Drawing for the job (mm, zero at the part's lowest x, y, z). A direction names the side the tool comes from. Round coordinates to 2 decimals unless told otherwise and drop trailing zeros. Loops run counter-clockwise (first coordinate to the right, second up) from the corner with the lowest first, then second, coordinate; pieces in that order, holes last.
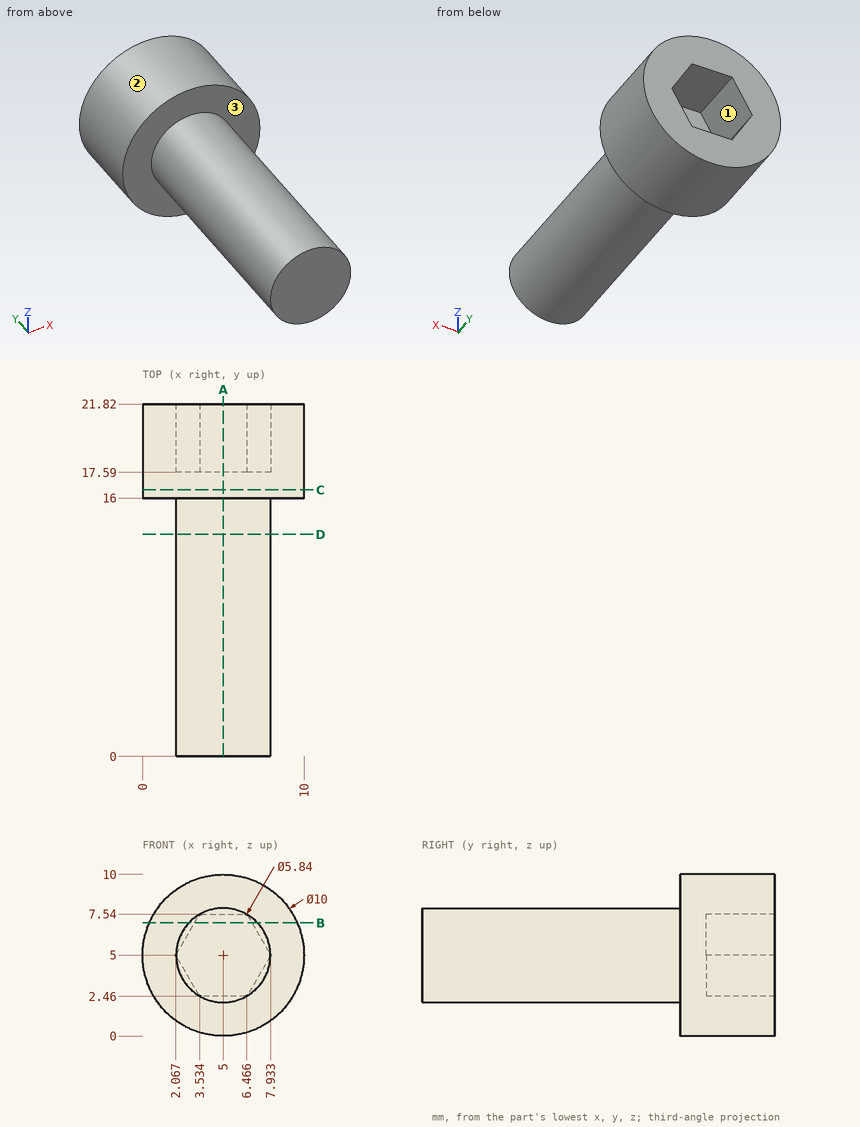
Q1. Probe line 1 (Z direction, x = 5, y = 20); line 2 (Y direction, x = 3, z = 9); line 3 (Y direction, x = 4.5, z = 3.5). List the from-to ranges inside material, lowest first.
Q2. Flat gauge pins, fed straight in: P1, Ø3, axis at y = 17, z = 3.5, coming from the -X side; P2, Ø1, axis at x = 2.5, y = 18.5, coming from the -Z side; P3, Ø2, axis at x = 7.5, z = 1.5, coming from the -Y side; P4, Ø6, axis at x = 3, y = 9.5, coming from the +Z side. Where does each tip first touch, or does it go through?
Q3. Slice it at C-C on y = 16.5. Give the cut face in (x, z).
Q4. Slice it at B-B on z = 7. Give the cut face in (x, y), plus the area to 3 significant figures.
Q5. Slice it at D-D on y = 13.75. Give the cut face in (x, z).
Q6. Tool access for the marked faces 1, 2 and 3: list every direction of +Z, -Z, +X, -X, +Y, -Y with a clear straight run to the whole face (end or side of a thin tool).
Q7. Slice it at A-A on x = 5. Give the cut face in (y, z).
Reply:
1. line 1: z = 0 to 2.46, 7.54 to 10
1. line 2: y = 16 to 21.82
1. line 3: y = 0 to 17.59
2. P1: stops at x = 0
2. P2: stops at z = 0.42
2. P3: stops at y = 16
2. P4: stops at z = 7.92
3. outline: circle Ø10 at (5, 5)
4. outline: (0.42, 16) - (2.87, 16) - (2.87, 0) - (7.13, 0) - (7.13, 16) - (9.58, 16) - (9.58, 21.82) - (6.78, 21.82) - (6.78, 17.59) - (3.22, 17.59) - (3.22, 21.82) - (0.42, 21.82) - close
4. area: 106 mm2
5. outline: circle Ø5.84 at (5, 5)
6. face 1: +Y
6. face 2: +Y, -Y
6. face 3: -Y
7. outline: (0, 2.08) - (16, 2.08) - (16, 0) - (21.82, 0) - (21.82, 2.46) - (17.59, 2.46) - (17.59, 7.54) - (21.82, 7.54) - (21.82, 10) - (16, 10) - (16, 7.92) - (0, 7.92) - close
